The model under review builds one solid part; all positions refer to its coordinate system, in mm. Round coordinates to 2 decimals unless told otherwise and drop trailing zeros. Write each loop counter-clockwise with the first axis right and the second up, starting at its lowest first coordinate (ties: lowest second). Pieces come first, ordered by that corner, then holes. Notation, with made-up numbers: (35.5, 30) -> (73.5, 30) arc R20 cw to (73.5, 45) -> close; hole circle Ø4 at (-31, 16). An arc over 180 degrees is marked (long way). Answer as a JSON object with one key per item and string values. Group by question number.
1) We need section B-B, the plane z = 14. Write out the cut boundary in (x, y).
2) We need section A-A, the plane y = -1. Write out the cut boundary in (x, z), then the cut area to 3 significant figures.
3) To check wall thickness, follow probe 1 along Y at (x, z) = (-33, 24); probe 2 along Y at (x, z) = (-69, -17); probe 3 along Z at (x, y) = (-44, -0.5). State the ranges of each line that lie inside material, in increasing order. Write a range as [from, to].
4) Insertion check: pin 1 Ø4.5 at (x, z) = (-71.69, -24.26) entering from -Y; pin 2 Ø5 at (x, z) = (-32.69, -24.26) entering from +Y; pin 3 Ø6 at (x, z) = (-71.5, 2.5) entering from +Y; pin 4 Ø4 at (x, y) = (-54, -2.5) entering from -Z. Each pin has a flat end and moves straight along its axis. Give the tip position at first contact, or say it passes through.
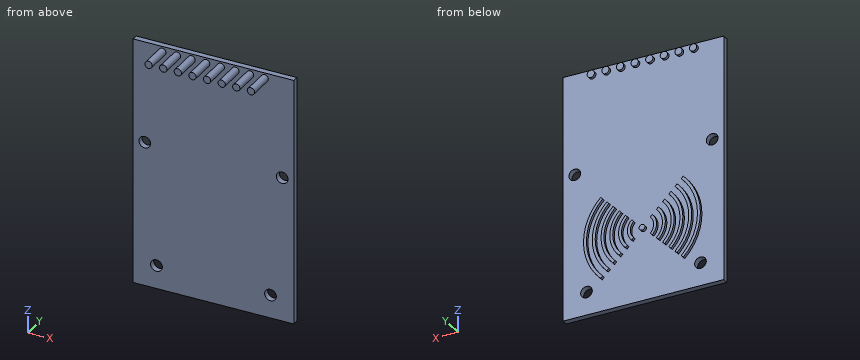
from build123d import *

# Parameters (mm, degrees)
ESBO_O1_W                     = 55
ESBO_O1_H                     = 85
RESSALTO_EXTRUS_O1_DEPTH      = 2
ESBO_O2_R                     = 1
RESSALTO_EXTRUS_O2_DEPTH      = 1
ESBO_O3_R                     = 1.25
RESSALTO_EXTRUS_O3_DEPTH      = 1
RESSALTO_EXTRUS_O3_DEPTH_BACK = 11
ESBO_O4_R                     = 2
CORTE_EXTRUS_O1_DEPTH         = 3


with BuildPart() as part:
    # Esboço1 → Ressalto-extrusão1 (new body)
    with BuildSketch(Plane(origin=(0, 0, 0), x_dir=(1, 0, 0), z_dir=(0, 1, 0))):
        with Locations((-52.185193749, -10.243624719)):
            Rectangle(ESBO_O1_W, ESBO_O1_H)
    extrude(amount=RESSALTO_EXTRUS_O1_DEPTH)

    # Esboço2 → Ressalto-extrusão2 (add)
    with BuildSketch(Plane(origin=(0, 2, 0), x_dir=(1, 0, 0), z_dir=(0, 1, 0))):
        with Locations((-52.185193749, 7.256375281)):
            Circle(ESBO_O2_R)
        with BuildLine():
            Line((-55.720727655, 10.791909187), (-55.013620874, 10.084802406))
            ThreePointArc((-55.013620874, 10.084802406), (-56.185193749, 7.256375281), (-55.013620874, 4.427948156))
            Line((-55.013620874, 4.427948156), (-55.720727655, 3.720841375))
            ThreePointArc((-55.720727655, 3.720841375), (-57.185193749, 7.256375281), (-55.720727655, 10.791909187))
        make_face()
        with BuildLine():
            Line((-57.842047999, 12.91322953), (-57.134941218, 12.206122749))
            ThreePointArc((-57.134941218, 12.206122749), (-59.185193749, 7.256375281), (-57.134941218, 2.306627813))
            Line((-57.134941218, 2.306627813), (-57.842047999, 1.599521031))
            ThreePointArc((-57.842047999, 1.599521031), (-60.185193749, 7.256375281), (-57.842047999, 12.91322953))
        make_face()
        with BuildLine():
            Line((-59.963368343, 15.034549874), (-59.256261561, 14.327443093))
            ThreePointArc((-59.256261561, 14.327443093), (-62.185193749, 7.256375281), (-59.256261561, 0.185307469))
            Line((-59.256261561, 0.185307469), (-59.963368343, -0.521799312))
            ThreePointArc((-59.963368343, -0.521799312), (-63.185193749, 7.256375281), (-59.963368343, 15.034549874))
        make_face()
        with BuildLine():
            Line((-62.084688686, 17.155870218), (-61.377581905, 16.448763436))
            ThreePointArc((-61.377581905, 16.448763436), (-65.185193749, 7.256375281), (-61.377581905, -1.936012875))
            Line((-61.377581905, -1.936012875), (-62.084688686, -2.643119656))
            ThreePointArc((-62.084688686, -2.643119656), (-66.185193749, 7.256375281), (-62.084688686, 17.155870218))
        make_face()
        with BuildLine():
            Line((-64.20600903, 19.277190561), (-63.498902248, 18.57008378))
            ThreePointArc((-63.498902248, 18.57008378), (-68.185193749, 7.256375281), (-63.498902248, -4.057333218))
            Line((-63.498902248, -4.057333218), (-64.20600903, -4.764439999))
            ThreePointArc((-64.20600903, -4.764439999), (-69.185193749, 7.256375281), (-64.20600903, 19.277190561))
        make_face()
        with BuildLine():
            Line((-66.327329373, 21.398510905), (-65.620222592, 20.691404123))
            ThreePointArc((-65.620222592, 20.691404123), (-71.185193749, 7.256375281), (-65.620222592, -6.178653562))
            Line((-65.620222592, -6.178653562), (-66.327329373, -6.885760343))
            ThreePointArc((-66.327329373, -6.885760343), (-72.185193749, 7.256375281), (-66.327329373, 21.398510905))
        make_face()
        with BuildLine():
            ThreePointArc((-49.356766625, 4.427948156), (-48.185193749, 7.256375281), (-49.356766625, 10.084802406))
            Line((-49.356766625, 10.084802406), (-48.649659844, 10.791909187))
            ThreePointArc((-48.649659844, 10.791909187), (-47.185193749, 7.256375281), (-48.649659844, 3.720841375))
            Line((-48.649659844, 3.720841375), (-49.356766625, 4.427948156))
        make_face()
        with BuildLine():
            ThreePointArc((-47.235446281, 2.306627813), (-45.185193749, 7.256375281), (-47.235446281, 12.206122749))
            Line((-47.235446281, 12.206122749), (-46.5283395, 12.91322953))
            ThreePointArc((-46.5283395, 12.91322953), (-44.185193749, 7.256375281), (-46.5283395, 1.599521031))
            Line((-46.5283395, 1.599521031), (-47.235446281, 2.306627813))
        make_face()
        with BuildLine():
            ThreePointArc((-45.114125938, 0.185307469), (-42.185193749, 7.256375281), (-45.114125938, 14.327443093))
            Line((-45.114125938, 14.327443093), (-44.407019156, 15.034549874))
            ThreePointArc((-44.407019156, 15.034549874), (-41.185193749, 7.256375281), (-44.407019156, -0.521799312))
            Line((-44.407019156, -0.521799312), (-45.114125938, 0.185307469))
        make_face()
        with BuildLine():
            ThreePointArc((-42.992805594, -1.936012875), (-39.185193749, 7.256375281), (-42.992805594, 16.448763436))
            Line((-42.992805594, 16.448763436), (-42.285698813, 17.155870218))
            ThreePointArc((-42.285698813, 17.155870218), (-38.185193749, 7.256375281), (-42.285698813, -2.643119656))
            Line((-42.285698813, -2.643119656), (-42.992805594, -1.936012875))
        make_face()
        with BuildLine():
            ThreePointArc((-40.87148525, -4.057333218), (-36.185193749, 7.256375281), (-40.87148525, 18.57008378))
            Line((-40.87148525, 18.57008378), (-40.164378469, 19.277190561))
            ThreePointArc((-40.164378469, 19.277190561), (-35.185193749, 7.256375281), (-40.164378469, -4.764439999))
            Line((-40.164378469, -4.764439999), (-40.87148525, -4.057333218))
        make_face()
        with BuildLine():
            ThreePointArc((-38.750164907, -6.178653562), (-33.185193749, 7.256375281), (-38.750164907, 20.691404123))
            Line((-38.750164907, 20.691404123), (-38.043058126, 21.398510905))
            ThreePointArc((-38.043058126, 21.398510905), (-32.185193749, 7.256375281), (-38.043058126, -6.885760343))
            Line((-38.043058126, -6.885760343), (-38.750164907, -6.178653562))
        make_face()
    extrude(amount=RESSALTO_EXTRUS_O2_DEPTH)

    # Esboço3 → Ressalto-extrusão3 (add, two sides)
    with BuildSketch(Plane(origin=(0, 2, 0), x_dir=(1, 0, 0), z_dir=(0, 1, 0))) as ressalto_extrus_o3_sk:
        with Locations((-69.685193749, -50.8911199)):
            Circle(ESBO_O3_R)
        with Locations((-64.685193749, -50.8911199)):
            Circle(ESBO_O3_R)
        with Locations((-59.685193749, -50.8911199)):
            Circle(ESBO_O3_R)
        with Locations((-54.685193749, -50.8911199)):
            Circle(ESBO_O3_R)
        with Locations((-49.685193749, -50.8911199)):
            Circle(ESBO_O3_R)
        with Locations((-44.685193749, -50.8911199)):
            Circle(ESBO_O3_R)
        with Locations((-39.685193749, -50.8911199)):
            Circle(ESBO_O3_R)
        with Locations((-34.685193749, -50.8911199)):
            Circle(ESBO_O3_R)
    extrude(amount=RESSALTO_EXTRUS_O3_DEPTH)
    extrude(ressalto_extrus_o3_sk.sketch, amount=-RESSALTO_EXTRUS_O3_DEPTH_BACK)

    # Esboço4 → Corte-extrusão1 (cut)
    with BuildSketch(Plane(origin=(0, 2, 0), x_dir=(1, 0, 0), z_dir=(0, 1, 0))):
        with Locations((-71.685193749, 24.256375281)):
            Circle(ESBO_O4_R)
        with Locations((-32.685193749, 24.256375281)):
            Circle(ESBO_O4_R)
        with Locations((-75.685193749, -17.743624719)):
            Circle(ESBO_O4_R)
        with Locations((-28.685193749, -17.743624719)):
            Circle(ESBO_O4_R)
    extrude(amount=-CORTE_EXTRUS_O1_DEPTH, mode=Mode.SUBTRACT)


solid = part.part
Here are the results:
{
 "1": {"outline": "(-79.69, 0) -> (-24.69, 0) -> (-24.69, 2) -> (-79.69, 2) -> close"},
 "2": {"outline": "circle Ø2.5 at (-69.69, 50.89); circle Ø2.5 at (-64.69, 50.89); circle Ø2.5 at (-59.69, 50.89); circle Ø2.5 at (-54.69, 50.89); circle Ø2.5 at (-49.69, 50.89); circle Ø2.5 at (-44.69, 50.89); circle Ø2.5 at (-39.69, 50.89); circle Ø2.5 at (-34.69, 50.89)", "area": "39.3 mm^2"},
 "3": {"probe 1": "y = [0, 2]", "probe 2": "y = [0, 3]", "probe 3": "z = [49.85, 51.94]"},
 "4": {"pin 1": "stops at y = 0", "pin 2": "stops at y = 2", "pin 3": "stops at y = 3", "pin 4": "stops at z = 49.64"}
}
